Source: CAD feature listing. Evaluate the final solid. Frame: model axes, mm. A direction names the side the tool comes from. Give positions to 0.01 mm unless a question says otherwise; leave off trailing zeros. Write each loop counter-clockwise with the first axis right and the second up, starting at its lowest first coordinate (ties: lowest second). Pieces come first, ordered by that corner, then holes. Notation, with made-up numbers: (-18.5, 56.5) -> (5.5, 56.5) arc R14 ccw to (5.5, 65.5) -> close; hole circle Ø6 at (77, 23.5). An arc over 180 degrees is marked (long way). Write item = value, one per line.
from build123d import *

# Parameters (mm, degrees)
BOX002_W      = 156
BOX002_H      = 72
BOX002_DEPTH  = 8
BOX001_W      = 10
BOX001_H      = 52
BOX001_DEPTH  = 10
BOX_W         = 160
BOX_H         = 72
BOX_DEPTH     = 10
SKETCH_R      = 1.65
HOLE_DEPTH    = 160.001
SKETCH001_R   = 1.65
HOLE001_DEPTH = 10.001
SKETCH002_R   = 1.375
HOLE002_DEPTH = 10.001
SKETCH003_R   = 1.65
HOLE003_DEPTH = 25


with BuildPart() as obj1:
    # Box002 → Box002 (new body)
    with BuildSketch(Plane(origin=(2, 0, 0), x_dir=(1, 0, 0), z_dir=(0, 0, 1))):
        with Locations((78, 36)):
            Rectangle(BOX002_W, BOX002_H)
    extrude(amount=BOX002_DEPTH)


with BuildPart() as obj2:
    # Box001 → Box001 (new body)
    with BuildSketch(Plane(origin=(0, 10, 0), x_dir=(1, 0, 0), z_dir=(0, 0, 1))):
        with Locations((5, 26)):
            Rectangle(BOX001_W, BOX001_H)
    extrude(amount=BOX001_DEPTH)


with BuildPart() as part_mirroring:
    # Part__Mirroring: instance of obj2
    add(obj2.part.mirror(Plane(origin=(80, 0, 0), x_dir=(0, -1, 0), z_dir=(1, 0, 0))))


with BuildPart() as body:
    # Box → Box (new body)
    with BuildSketch(Plane.XY):
        with Locations((80, 36)):
            Rectangle(BOX_W, BOX_H)
    extrude(amount=BOX_DEPTH)

    # Cut: cut obj2
    add(obj2.part, mode=Mode.SUBTRACT)

    # Cut001: cut Part__Mirroring
    add(part_mirroring.part, mode=Mode.SUBTRACT)

    # Cut002: cut obj1
    add(obj1.part, mode=Mode.SUBTRACT)

    # Sketch (on Face1 of BaseFeature) → Hole (cut, through all)
    with BuildSketch(Plane(origin=(0, 0, 0), x_dir=(0, -1, 0), z_dir=(-1, 0, 0))):
        with Locations((-5, 4)):
            Circle(SKETCH_R)
        with Locations((-67, 4)):
            Circle(SKETCH_R)
    extrude(amount=-HOLE_DEPTH, mode=Mode.SUBTRACT)

    # Sketch001 (on Face2 of Hole) → Hole001 (cut, through all)
    with BuildSketch(Plane.XY.offset(10)):
        with Locations((72.25, 40.25)):
            Circle(SKETCH001_R)
        with Locations((87.75, 40.25)):
            Circle(SKETCH001_R)
        with Locations((128, 69)):
            Circle(SKETCH001_R)
        with Locations((128, 3)):
            Circle(SKETCH001_R)
    extrude(amount=-HOLE001_DEPTH, mode=Mode.SUBTRACT)

    # Sketch002 (on Face2 of Hole) → Hole002 (cut, through all)
    with BuildSketch(Plane.XY.offset(10)):
        with Locations((25, 60.5)):
            Circle(SKETCH002_R)
        with Locations((83, 60.5)):
            Circle(SKETCH002_R)
        with Locations((25, 11.5)):
            Circle(SKETCH002_R)
        with Locations((83, 11.5)):
            Circle(SKETCH002_R)
    extrude(amount=-HOLE002_DEPTH, mode=Mode.SUBTRACT)

    # Sketch003 (on Face2 of Hole002) → Hole003 (cut)
    with BuildSketch(Plane.XY.offset(10)):
        with Locations((69.5, 5)):
            Circle(SKETCH003_R)
        with Locations((90.5, 5)):
            Circle(SKETCH003_R)
    extrude(amount=-HOLE003_DEPTH, mode=Mode.SUBTRACT)


solid = body.part
1) Cut plane A-A (y = 37). Return the cut outline in (x, z).
Computed:
outline = (10, 8) -> (150, 8) -> (150, 10) -> (10, 10) -> close
2) Material intervals for L1, parallel to Y at x = 25, z = 8.75 (3 decimals); L2, parallel to Z at x = 0.6, y = 5; L3, parallel to Y at x = 87.75, z = 9.25, sorted ascending.
Computed:
L1 = 0 to 10.125, 12.875 to 59.125, 61.875 to 72
L2 = 0 to 2.35, 5.65 to 10
L3 = 0 to 38.6, 41.9 to 72
3) Draft query along Y for faces 1 (the flat face through (158, 5, 6)), 2 (the flat face through (1.6, 62, 7.2)), 3 (the flat face through (80, 72, 9)). Return one class per face: pulls with the +Y half, pulls with the -Y half, needs draft (parallel to the pull), parting line crosses it, or undercut.
Computed:
face_1 = needs draft
face_2 = undercut
face_3 = pulls with the +Y half
4) Cut plane B-B (x = 136). Return the cut outline in (y, z), then the cut area to 3 significant figures.
Computed:
outline = (0, 8) -> (72, 8) -> (72, 10) -> (0, 10) -> close
area = 144 mm²
5) Access query for faces 4 (the flat face through (158.4, 10, 7.2)), 5 (the flat face through (1.6, 10, 7.2)), 6 (the flat face through (2, 67, 6)), 7 (the cylindrical face through (129.524, 68.368, 9.014)). Directions: +Z, -Z, +X, -X, +Y, -Y. A direction counts if a zero-diameter tool reaches every point of the face in a straight line with its end or side. Return the directions, or none.
Computed:
face_4 = +Z, -Z, +X
face_5 = +Z, -Z, -X
face_6 = -Z, +Y, -Y
face_7 = +Z, -Z
6) Contact query for flat-ended pins moving along their axis: pin 1 (8 mm diameter, centred on x = 113, y = 57, fed in from -Z); pin 2 (3 mm diameter, centred on x = 155, z = 5.5, fed in from +Y); pin 3 (6 mm diameter, centred on y = 12.5, z = 8, fed in from -X). Output: stop coordinate, or through.
Computed:
pin_1 = 8
pin_2 = through
pin_3 = 0
